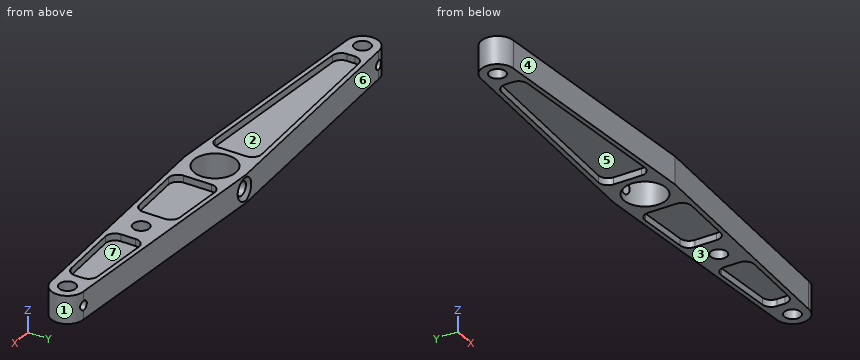
from build123d import *

# Parameters (mm, degrees)
SKETCH1_R           = 4.5
SKETCH1_R_2         = 1.75
BOSS_EXTRUDE1_DEPTH = 6
CUT_EXTRUDE1_DEPTH  = 1.5
LPATTERN1_COUNT     = 2
LPATTERN1_PITCH     = 4.5
CUT_EXTRUDE2_DEPTH  = 1.5
LPATTERN2_COUNT     = 2
LPATTERN2_PITCH     = 4.5
CUT_EXTRUDE3_DEPTH  = 1.5
LPATTERN3_COUNT     = 2
LPATTERN3_PITCH     = 4.5
SKETCH5_R           = 1.75
CUT_EXTRUDE4_DEPTH  = 11.5
SKETCH8_R           = 1
CUT_EXTRUDE5_DEPTH  = 7


with BuildPart() as part:
    # Sketch1 → Boss-Extrude1 (new body)
    with BuildSketch(Plane.XY):
        with BuildLine():
            Line((0, -6.5), (51, -3.5))
            ThreePointArc((51, -3.5), (54.5, 0), (51, 3.5))
            Line((51, 3.5), (-0.383128511, 6.488698833))
            Line((-0.383128511, 6.488698833), (-51, 3.5))
            ThreePointArc((-51, 3.5), (-54.5, 0), (-51, -3.5))
            Line((-51, -3.5), (0, -6.5))
        make_face()
        Circle(SKETCH1_R, mode=Mode.SUBTRACT)
        with Locations((-51, 0)):
            Circle(SKETCH1_R_2, mode=Mode.SUBTRACT)
        with Locations((51, 0)):
            Circle(SKETCH1_R_2, mode=Mode.SUBTRACT)
    extrude(amount=BOSS_EXTRUDE1_DEPTH)

    # Sketch2 → Cut-Extrude1 (cut)
    with BuildSketch(Plane.XY.offset(6)):
        with BuildLine():
            Line((-8.117885696, 5.030254505), (-45.117885696, 2.845570751))
            ThreePointArc((-45.117885696, 2.845570751), (-46.455295742, 2.220949744), (-47, 0.849048033))
            Line((-47, 0.849048033), (-47, -0.847755347))
            ThreePointArc((-47, -0.847755347), (-46.455143994, -2.219818012), (-45.117444044, -2.844304094))
            Line((-45.117444044, -2.844304094), (-8.117444044, -5.020774682))
            ThreePointArc((-8.117444044, -5.020774682), (-6.627937335, -4.47936993), (-6, -3.024225935))
            Line((-6, -3.024225935), (-6, 3.033731787))
            ThreePointArc((-6, 3.033731787), (-6.628098289, 4.489027529), (-8.117885696, 5.030254505))
        make_face()
    cut_extrude1 = extrude(amount=-CUT_EXTRUDE1_DEPTH, mode=Mode.SUBTRACT)

    # LPattern1: Cut-Extrude1 ×2
    with Locations(*[(0, 0, -i * LPATTERN1_PITCH) for i in range(1, LPATTERN1_COUNT)]):
        add(cut_extrude1, mode=Mode.SUBTRACT)

    # Sketch3 → Cut-Extrude2 (cut)
    with BuildSketch(Plane.XY.offset(6)):
        with BuildLine():
            Line((8.116133684, 4.992649231), (19.116133684, 4.352834411))
            ThreePointArc((19.116133684, 4.352834411), (20.454693673, 3.728749112), (21, 2.356209016))
            Line((21, 2.356209016), (21, -2.377167112))
            ThreePointArc((21, -2.377167112), (20.455143994, -3.749229777), (19.117444044, -4.373715858))
            Line((19.117444044, -4.373715858), (8.117444044, -5.020774682))
            ThreePointArc((8.117444044, -5.020774682), (6.627937335, -4.47936993), (6, -3.024225935))
            Line((6, -3.024225935), (6, 2.996023836))
            ThreePointArc((6, 2.996023836), (6.627459904, 4.45071751), (8.116133684, 4.992649231))
        make_face()
    cut_extrude2 = extrude(amount=-CUT_EXTRUDE2_DEPTH, mode=Mode.SUBTRACT)

    # LPattern2: Cut-Extrude2 ×2
    with Locations(*[(0, 0, -i * LPATTERN2_PITCH) for i in range(1, LPATTERN2_COUNT)]):
        add(cut_extrude2, mode=Mode.SUBTRACT)

    # Sketch4 → Cut-Extrude3 (cut)
    with BuildSketch(Plane.XY.offset(6)):
        with BuildLine():
            Line((47, 0.843919439), (47, -0.847755347))
            ThreePointArc((47, -0.847755347), (46.455143994, -2.219818012), (45.117444044, -2.844304094))
            Line((45.117444044, -2.844304094), (32.117444044, -3.609009976))
            ThreePointArc((32.117444044, -3.609009976), (30.627937335, -3.067605224), (30, -1.61246123))
            Line((30, -1.61246123), (30, 1.600064227))
            ThreePointArc((30, 1.600064227), (30.627459904, 3.054757901), (32.116133684, 3.596689622))
            Line((32.116133684, 3.596689622), (45.116133684, 2.840544834))
            ThreePointArc((45.116133684, 2.840544834), (46.454693673, 2.216459536), (47, 0.843919439))
        make_face()
    cut_extrude3 = extrude(amount=-CUT_EXTRUDE3_DEPTH, mode=Mode.SUBTRACT)

    # LPattern3: Cut-Extrude3 ×2
    with Locations(*[(0, 0, -i * LPATTERN3_PITCH) for i in range(1, LPATTERN3_COUNT)]):
        add(cut_extrude3, mode=Mode.SUBTRACT)

    # Sketch5 → Cut-Extrude4 (cut)
    with BuildSketch(Plane.XY.offset(6)):
        with Locations((25.5, 0)):
            Circle(SKETCH5_R)
    extrude(amount=-CUT_EXTRUDE4_DEPTH, mode=Mode.SUBTRACT)

    # Sketch7 → Cut-Revolve1 (revolve, cut)
    with BuildSketch(Plane(origin=(0, 0, 0), x_dir=(0, 0, -1), z_dir=(1, 0, 0)), mode=Mode.PRIVATE) as cut_revolve1_sk:
        Polygon((-3, 6.488698833), (-5.5, 6.488698833), (-4.5, 5.75735408), (-4.5, 2.301697652), (-3, 2.301697652), (-3, 5.75735408), align=None)
    revolve(cut_revolve1_sk.sketch.rotate(Axis((0, 2.301697652, 3), (0, 1, 0)), 351.184602487), axis=Axis((0, 2.301697652, 3), (0, 1, 0)), mode=Mode.SUBTRACT)

    # Sketch8 → Cut-Extrude5 (cut)
    with BuildSketch(Plane(origin=(0, 6.488698833, 0), x_dir=(1, 0, 0), z_dir=(0, 1, 0))):
        with Locations(Location((-51, -3, 0), (0, 0, 270))):
            Circle(SKETCH8_R)
        with Locations(Location((51, -3, 0), (0, 0, 270))):
            Circle(SKETCH8_R)
    extrude(amount=-CUT_EXTRUDE5_DEPTH, mode=Mode.SUBTRACT)


solid = part.part
Geometry: final body of the model. Coordinates: model frame, mm. Face numbers are marked on the shaded views. A direction names the side the tool comes from. Round coordinates to 2 decimals unless told otherwise and drop trailing zeros. Loops run counter-clockwise (first coordinate to the right, second up) from the corner with the lowest first, then second, coordinate; pieces in that order, holes last.
Q1. Access query for the marked faces 5, 6 and 7. Directions: +Z, -Z, +X, -X, +Y, -Y. A direction counts if a zero-diameter tool reaches every point of the face in a straight line with its end or side. Return the directions, or none.
Q2. Material intervals for L1, parallel to Y at x = 25.5, z = 3.1; L2, parallel to Z at x = 51, y = 2; L3, parallel to X at y = -0.5, z = 2, sorted ascending.
Q3. Section B-B on z = 3. Return loops of the section in (x, y).
Q4. Section D-D on x = -44. Return loops of the section in (y, z), plus the area to 3 significant figures.
Q5. Pull-direction query (Y, two-part tool) for the marked faces 1, 2, 3 and 4; classes: released by +Y, released by -Y, zero draft, split by the parting line, or undercut.
Q6. Section C-C on x = -27. Return loops of the section in (y, z).
Q7. Section A-A on x = 25.5. Return loops of the section in (y, z).
Q8. Pin query (flat end, axial travel): P1, Ø2, axis at x = -51, y = 0, coming from the -Z side; P2, Ø1.8, axis at x = -51, z = 3, coming from the -Y side; P3, Ø1.6, axis at y = -1, z = 5, coming from the -X side; P4, Ø0.8, axis at y = 1.5, z = 0.5, coming from the +X side. Return the tip coordinate at first contact, or that it passes through.
Evaluation:
1. face 5: -Z
1. face 6: +Z, -Z, -X, +Y
1. face 7: +Z
2. L1: y = -5 to -1.75, 1.75 to 4.98
2. L2: z = 0 to 2, 4 to 6
2. L3: x = -54.46 to -52.68, -49.32 to -4.47, 4.47 to 23.82, 27.18 to 49.32, 52.68 to 54.46
3. outline: (-52, 1.44) - (-52, 3.35) arc R3.5 ccw to (-51, -3.5) - (0, -6.5) - (51, -3.5) arc R3.5 ccw to (52, 3.35) - (52, 1.44) arc R1.75 cw (long way) to (50, 1.44) - (50, 3.56) - (2.29, 6.33) - (1.5, 5.76) - (1.5, 4.24) arc R4.5 cw (long way) to (-1.5, 4.24) - (-1.5, 5.76) - (-2.34, 6.37) - (-50, 3.56) - (-50, 1.44) arc R1.75 cw (long way) to start; hole circle Ø3.5 at (25.5, 0)
4. outline: (-3.91, 0) - (-2.91, 0) - (-2.91, 1.5) - (2.91, 1.5) - (2.91, 0) - (3.91, 0) - (3.91, 6) - (2.91, 6) - (2.91, 4.5) - (-2.91, 4.5) - (-2.91, 6) - (-3.91, 6) - close
4. area: 29.5 mm2
5. face 1: split by the parting line
5. face 2: undercut
5. face 3: zero draft
5. face 4: released by -Y
6. outline: (-4.91, 0) - (-3.91, 0) - (-3.91, 1.5) - (3.92, 1.5) - (3.92, 0) - (4.92, 0) - (4.92, 6) - (3.92, 6) - (3.92, 4.5) - (-3.91, 4.5) - (-3.91, 6) - (-4.91, 6) - close
7. outline: (-5, 0) - (-1.75, 0) - (-1.75, 6) - (-5, 6) - close; (1.75, 0) - (4.98, 0) - (4.98, 6) - (1.75, 6) - close
8. P1: passes through
8. P2: stops at y = -3.55
8. P3: stops at x = -54.49
8. P4: stops at x = 54.32
